from build123d import *

# Parameters (mm, degrees)
CROQUIS1_W                 = 90
CROQUIS1_H                 = 50
SALIENTE_EXTRUIR1_DEPTH    = 100
REDONDEO1_R                = 25
CORTAR_EXTRUIR1_DEPTH      = 25
CORTAR_EXTRUIR1_DEPTH_BACK = 25
CROQUIS2_W                 = 30
CROQUIS2_H                 = 40
CROQUIS4_R                 = 10
CORTAR_EXTRUIR2_DEPTH      = 100
CROQUIS3_W                 = 40
CROQUIS3_H                 = 20
CORTAR_EXTRUIR3_DEPTH      = 50
CROQUIS5_R                 = 10
CORTAR_EXTRUIR4_DEPTH      = 20


with BuildPart() as part:
    # Croquis1 → Saliente-Extruir1 (new body)
    with BuildSketch(Plane.XY):
        Rectangle(CROQUIS1_W, CROQUIS1_H)
    extrude(amount=SALIENTE_EXTRUIR1_DEPTH)

    # Redondeo1
    redondeo1_edges = [part.edges().sort_by_distance(p)[0] for p in [
        (45, -25, 50),
        (45, 25, 50),
        (-45, -25, 50),
        (-45, 25, 50),
    ]]
    fillet(redondeo1_edges, radius=REDONDEO1_R - 0.0001)  # a hair under: the kernel refuses the full size

    # Croquis2 → Cortar-Extruir1 (cut, two sides: drawn at the far end of the back side and taken through both)
    with BuildSketch(Plane(origin=(0, 0, 0), x_dir=(1, 0, 0), z_dir=(0, 1, 0)).offset(-CORTAR_EXTRUIR1_DEPTH_BACK)):
        with Locations((30, -20)):
            Rectangle(CROQUIS2_W, CROQUIS2_H)
        with Locations((30, -80)):
            Rectangle(CROQUIS2_W, CROQUIS2_H)
    extrude(amount=CORTAR_EXTRUIR1_DEPTH + CORTAR_EXTRUIR1_DEPTH_BACK, mode=Mode.SUBTRACT)

    # Croquis4 → Cortar-Extruir2 (cut)
    with BuildSketch(Plane.XY.offset(100)):
        with Locations((-20, 0)):
            Circle(CROQUIS4_R)
    extrude(amount=-CORTAR_EXTRUIR2_DEPTH, mode=Mode.SUBTRACT)

    # Croquis3 → Cortar-Extruir3 (cut)
    with BuildSketch(Plane(origin=(0, 25, 0), x_dir=(1, 0, 0), z_dir=(0, 1, 0))):
        with Locations((-25, -50)):
            Rectangle(CROQUIS3_W, CROQUIS3_H)
    extrude(amount=-CORTAR_EXTRUIR3_DEPTH, mode=Mode.SUBTRACT)

    # Croquis5 → Cortar-Extruir4 (cut)
    with BuildSketch(Plane.XY.offset(60)):
        with Locations((30, 0)):
            Circle(CROQUIS5_R)
    extrude(amount=-CORTAR_EXTRUIR4_DEPTH, mode=Mode.SUBTRACT)


solid = part.part
The listing builds one solid part. Answer for the finished solid, in the listing's coordinates (mm). A direction names the side the tool comes from. Round coordinates to 2 decimals unless told otherwise and drop trailing zeros. Order: outer loops, then holes, each group sorted by start corner. A loop starts at its lowest first (then second) coordinate and runs counter-clockwise, first axis right, second up. Notation, with made-up numbers: (41.25, -21.75) -> (69.25, -21.75) arc R34 cw to (69.25, 9.25) -> close; hole circle Ø1 at (67.25, 50.5). An arc over 180 degrees is marked (long way). Put each result on its own line as item: value.
Q1. Section D-D, the plane x = -22.5 is taken. Write down the section's boundary in (y, z).
Results list:
outline: (-24.87, 0) -> (-9.68, 0) -> (-9.68, 40) -> (-24.87, 40) -> close; (-24.87, 60) -> (-9.68, 60) -> (-9.68, 100) -> (-24.87, 100) -> close; (9.68, 0) -> (24.87, 0) -> (24.87, 40) -> (9.68, 40) -> close; (9.68, 60) -> (24.87, 60) -> (24.87, 100) -> (9.68, 100) -> close
Q2. Each of these flat-tipped pins is pushed along its axis until it touches: P1, Ø2, axis at y = 3, z = 66.5, coming from the +X side; P2, Ø4, axis at y = -16, z = 47.5, coming from the +X side; P3, Ø6, axis at y = 3.5, z = 46.5, coming from the -X side. Where does it stop, or does it pass through?
Results list:
P1: x = 15
P2: x = 40.71
P3: x = -5
Q3. Consider line 1 along Z through (x, y) = (-37.5, 1.5); line 2 along Y through (x, z) = (-20, 75); line 3 along Z through (x, y) = (40, 2.5). Determine where each line is inside the solid, lowest interval first.
Results list:
line 1: 0 to 40, 60 to 100
line 2: -25 to -10, 10 to 25
line 3: 40 to 60
Q4. Which of the six approach directions +Z, -Z, +X, -X, +Y, -Y give full straight-line access (tool end or side, diameter ignored) to faces 1 (the flat face through (19.8, -0.4, 40)), 2 (the cylindrical face through (-37.871, -17.482, 80.28)), 3 (the flat face through (-30, -5, 60)), 4 (the flat face through (15, 0, 80))?
Results list:
face 1: -Z, +X, +Y, -Y
face 2: +Z, -Z, -X, -Y
face 3: -X, +Y, -Y
face 4: +Z, +X, +Y, -Y
Q5. Determine the mould class of faces 5 (the flat face through (19.8, -0.4, 60)), 6 (the cylindrical face through (-10.46, 3, 20.28)), 7 (the cylindrical face through (39.54, 3, 50.14)), 8 (the cylindrical face through (37.482, -17.871, 50.14)) for opening direction X: pulls with the +X half, pulls with the -X half, needs draft (parallel to the pull), parting line crosses it, or undercut.
Results list:
face 5: needs draft
face 6: undercut
face 7: undercut
face 8: pulls with the +X half
Q6. Section B-B, the plane x = -39 is taken. Write down the section's boundary in (y, z), and give its area (3 significant figures).
Results list:
outline: (-16.25, 0) -> (16.25, 0) -> (16.25, 40) -> (-16.25, 40) -> close; (-16.25, 60) -> (16.25, 60) -> (16.25, 100) -> (-16.25, 100) -> close
area: 2,600 mm^2
Q7. Section C-C, the plane y = -19 is taken. Write down the section's boundary in (x, z).
Results list:
outline: (-36.25, 0) -> (15, 0) -> (15, 40) -> (36.25, 40) -> (36.25, 60) -> (15, 60) -> (15, 100) -> (-36.25, 100) -> (-36.25, 60) -> (-5, 60) -> (-5, 40) -> (-36.25, 40) -> close
